The model under review builds one solid part; all positions refer to its coordinate system, in mm. Face numbers are marked on the shaded views. A direction names the side the tool comes from. Coordinates: 2 decimals unless noted, no trailing zeros. Order: outer loops, then holes, each group sorted by start corner. A loop starts at its lowest first (then second) coordinate and runs counter-clockwise, first axis right, second up. Notation, with made-up numbers: (40.25, 47.5) -> (92.25, 47.5) arc R22 ccw to (92.25, 80.5) -> close; hole circle Ø9 at (13.25, 35). An arc over 180 degrees is marked (long way). Answer as CSV lines item,"result". Start each with the question number.
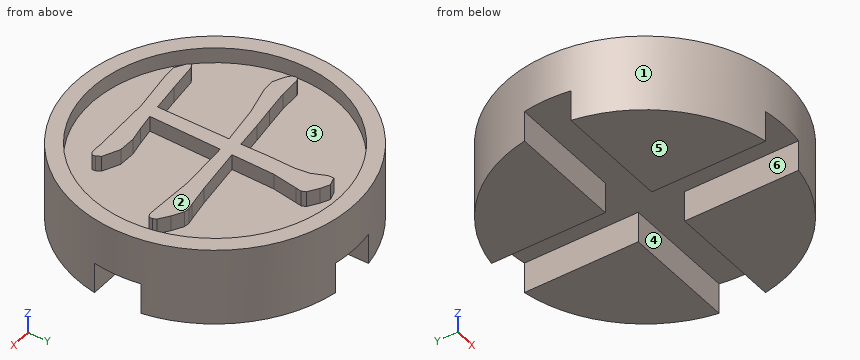
from build123d import *

# Parameters (mm, degrees)
F0_R     = 9
F1_DEPTH = 4
F3_W     = 3
F3_H     = 3
F4_DEPTH = 2
F2_R     = 9
F2_R_2   = 8
F5_DEPTH = 1
F7_DEPTH = 1


# Not quite as in the source:
# - a feature names something its author has since deleted; it is built from what else it names


with BuildPart() as f1:
    # F0 (on Top) → F1 (new body)
    with BuildSketch(Plane.XY):
        with Locations((-31.3306450844, 19.7580661625)):
            Circle(F0_R)
    extrude(amount=F1_DEPTH)

    # F3 (on face) → F4 (cut)
    with BuildSketch(Plane(origin=(0, 0, 0), x_dir=(1, 0, 0), z_dir=(0, 0, -1))):
        with BuildLine():
            ThreePointArc((-32.8306450844, -28.6321858371), (-32.0832814269, -28.7265408676), (-31.3306450844, -28.7580661625))
            ThreePointArc((-31.3306450844, -28.7580661625), (-30.5780087419, -28.7265408676), (-29.8306450844, -28.6321858371))
            Line((-29.8306450844, -28.6321858371), (-29.8306450844, -21.2580661625))
            Line((-29.8306450844, -21.2580661625), (-32.8306450844, -21.2580661625))
            Line((-32.8306450844, -21.2580661625), (-32.8306450844, -28.6321858371))
        make_face()
        with BuildLine():
            ThreePointArc((-40.204764759, -18.2580661625), (-40.2991197895, -19.0054298199), (-40.3306450844, -19.7580661625))
            ThreePointArc((-40.3306450844, -19.7580661625), (-40.2991197895, -20.510702505), (-40.204764759, -21.2580661625))
            Line((-40.204764759, -21.2580661625), (-32.8306450844, -21.2580661625))
            Line((-32.8306450844, -21.2580661625), (-32.8306450844, -18.2580661625))
            Line((-32.8306450844, -18.2580661625), (-40.204764759, -18.2580661625))
        make_face()
        with Locations((-31.3306450844, -19.7580661625)):
            Rectangle(F3_W, F3_H)
        with BuildLine():
            Line((-29.8306450844, -18.2580661625), (-29.8306450844, -21.2580661625))
            Line((-29.8306450844, -21.2580661625), (-22.4565254097, -21.2580661625))
            ThreePointArc((-22.4565254097, -21.2580661625), (-22.3621703793, -20.510702505), (-22.3306450844, -19.7580661625))
            ThreePointArc((-22.3306450844, -19.7580661625), (-22.3621703793, -19.0054298199), (-22.4565254097, -18.2580661625))
            Line((-22.4565254097, -18.2580661625), (-29.8306450844, -18.2580661625))
        make_face()
        with BuildLine():
            Line((-32.8306450844, -10.8839464878), (-32.8306450844, -18.2580661625))
            Line((-32.8306450844, -18.2580661625), (-29.8306450844, -18.2580661625))
            Line((-29.8306450844, -18.2580661625), (-29.8306450844, -10.8839464878))
            ThreePointArc((-29.8306450844, -10.8839464878), (-30.5780087419, -10.7895914574), (-31.3306450844, -10.7580661625))
            ThreePointArc((-31.3306450844, -10.7580661625), (-32.0832814269, -10.7895914574), (-32.8306450844, -10.8839464878))
        make_face()
    extrude(amount=-F4_DEPTH, mode=Mode.SUBTRACT)

    # F2 (on face) → F5 (join)
    with BuildSketch(Plane.XY.offset(4)):
        with Locations((-31.3306450844, 19.7580661625)):
            Circle(F2_R)
        with Locations((-31.3306450844, 19.7580661625)):
            Circle(F2_R_2, mode=Mode.SUBTRACT)
    extrude(amount=F5_DEPTH)

    # F6 (on face) → F7 (join)
    with BuildSketch(Plane.XY.offset(4)):
        Polygon((-32.0563357805, 20.1492391588), (-32.0563357805, 15.5241883096), (-33.8901808177, 15.2807091812), (-35.7654903866, 15.0600261471), (-36.0265778437, 14.9108290182), (-35.8773882333, 14.6911827853), (-35.2526459317, 14.3130134752), (-34.3978675811, 14.3513488068), (-31.6491488168, 14.7523119557), (-27.7544977602, 14.8984009364), (-27.2406082337, 14.8818211386), (-26.9360337682, 14.9129041244), (-26.7764911822, 15.0434478529), (-26.7972422443, 15.2371920988), (-26.9670851763, 15.5241883096), (-28.0156152913, 16.0142517072), (-29.0890316438, 16.0380853546), (-30.0566626908, 15.8391533431), (-31.1736036441, 15.6526644505), (-31.0741413977, 20.2777152997), (-27.8239687071, 20.5025335092), (-24.8161924809, 20.3896206649), (-24.4701910762, 20.3927258057), (-24.2691463661, 20.5014959561), (-24.248470489, 20.7273742743), (-24.368616131, 20.9532450739), (-25.0037038896, 21.403934083), (-25.6989396543, 21.7862799203), (-26.0398284784, 21.8225190939), (-26.4241742369, 21.7406426207), (-27.8850941182, 21.4816227513), (-31.057540548, 21.0485495894), (-31.0016029024, 23.7941707314), (-30.738440339, 25.4290687202), (-30.678367518, 25.7761979), (-30.788137629, 26.0549087229), (-31.4533219461, 26.4797040154), (-32.0066084166, 26.7469867172), (-32.5702328255, 26.5687982493), (-32.5702328255, 26.2164813041), (-32.1775490497, 25.3202760143), (-32.0563357805, 24.3681330789), (-32.0874247812, 22.6793274398), (-32.0563357805, 20.9200960041), (-33.8093644531, 20.709758427), (-35.2516083786, 20.5014959561), (-36.7901718172, 20.2932635593), (-38.0780173149, 20.2445662299), (-38.2831611116, 20.1761854655), (-38.351541876, 20.0373337936), (-38.2738359152, 19.7938772208), (-38.0117086494, 19.5731716311), (-37.2781676271, 19.2260875624), (-36.4534482425, 19.2830853166), (-34.5957620394, 19.7586530447), align=None)
    extrude(amount=F7_DEPTH)


solid = f1.part
1) Consider section C-C (z = 4.3). Count the separate pieces of the cut face and the enclosed holes in it, plus the area to 3 significant figures.
2) Wall thickness on L1, parallel to Y at x = -37.5, z = 4.45; L2, parallel to Z at x = -28.25, y = 23.5; L3, parallel to X at y = 16.25, z = 0.3: over which ranges is each line inside the solid? List them lowest first. Write a range as [from, to].
3) Tool access review of the marked faces 4, 5 and 6: name each direction out of +Z, -Z, +X, -X, +Y, -Y from which nothing blocks a thin tool from reaching the whole face with its end or side.
4) Consider section A-A (z = 1.15). Give the boundary of the cut face in (x, y), plus the area to 3 significant figures.
5) Consider section D-D (y = 17). Give the boundary of the cut face in (x, z), plus the area to 3 significant figures.
6) Consider section B-B (y = 27.5). Give the boundary of the cut face in (x, z).
7) Insertion check: pin 1 Ø1.6 at (x, z) = (-26, 1.5) entering from -Y; pin 2 Ø1.1 at (y, z) = (19, 4.5) entering from -X; pin 3 Ø2 at (y, z) = (23.5, 0.5) entering from -X. Each pin has a flat end and moves straight along its axis. Give the tip position at first contact, or say it passes through.
8) Mouldability with a two-part tool opening along X and no side actions: class the marked faces 1, 2 and 3 as released by +X, released by -X, zero draft, split by the parting line, or undercut.
Result:
1,separate pieces,"2"
1,enclosed holes,"1"
1,area,"85.7 mm2"
2,L1,"[13.21, 14.67], [19.33, 20.27], [24.85, 26.31]"
2,L2,"[0, 4]"
2,L3,"[-39.62, -32.83], [-29.83, -23.04]"
3,face 4,"-Z, +X, -X"
3,face 5,"-Z, +X, -X, +Y, -Y"
3,face 6,"-Z, +Y, -Y"
4,outline,"(-40.2, 18.26) arc R9 ccw to (-32.83, 10.88) -> (-32.83, 18.26) -> close; (-40.2, 21.26) -> (-32.83, 21.26) -> (-32.83, 28.63) arc R9 ccw to start; (-29.83, 10.88) arc R9 ccw to (-22.46, 18.26) -> (-29.83, 18.26) -> close; (-29.83, 21.26) -> (-22.46, 21.26) arc R9 ccw to (-29.83, 28.63) -> close"
4,area,"156 mm2"
5,outline,"(-39.9, 0) -> (-32.83, 0) -> (-32.83, 2) -> (-29.83, 2) -> (-29.83, 0) -> (-22.76, 0) -> (-22.76, 5) -> (-23.82, 5) -> (-23.82, 4) -> (-31.14, 4) -> (-31.14, 5) -> (-32.06, 5) -> (-32.06, 4) -> (-38.84, 4) -> (-38.84, 5) -> (-39.9, 5) -> close"
5,area,"65.6 mm2"
6,outline,"(-35.92, 0) -> (-32.83, 0) -> (-32.83, 2) -> (-29.83, 2) -> (-29.83, 0) -> (-26.74, 0) -> (-26.74, 5) -> (-29.32, 5) -> (-29.32, 4) -> (-33.35, 4) -> (-33.35, 5) -> (-35.92, 5) -> close"
7,pin 1,"y = 11.98"
7,pin 2,"x = -40.33"
7,pin 3,"x = -39.9"
8,face 1,"split by the parting line"
8,face 2,"zero draft"
8,face 3,"undercut"
